Here's how the part is built. I have some questions about the finished solid (model axes, mm). A direction names the side the tool comes from. Round coordinates to 2 decimals unless told otherwise and drop trailing zeros. Order: outer loops, then holes, each group sorted by start corner. A loop starts at its lowest first (then second) coordinate and runs counter-clockwise, first axis right, second up. Notation, with made-up numbers: M 9,87.5 L 24,87.5 A18 ccw 24,122.5 Z; hole C 70.5,11 d1. An arc over 180 degrees is marked long. Use one line per item in the form item = value. Start each with the question number.
```python
from build123d import *

# Parameters (mm, degrees)
SKETCH1_W           = 12.7
SKETCH1_H           = 12.7
BOSS_EXTRUDE1_DEPTH = 2.54
FILLET1_R           = 0.635
SHELL1_START        = 0.635
SHELL1_OUTLINE_W    = 1.905
SHELL1_OUTLINE_H    = 11.43
SHELL1_DEPTH        = 11.43
SKETCH2_R           = 2.54
BOSS_EXTRUDE2_DEPTH = 1.905
BOSS_EXTRUDE3_DEPTH = 0.00254


# Read off the part's stored shape, not the designer's step: Shell1
with BuildPart() as part:
    # Sketch1 → Boss-Extrude1 (new body)
    with BuildSketch(Plane(origin=(0, 0, 0), x_dir=(1, 0, 0), z_dir=(0, 1, 0))):
        with Locations((6.35, 6.35)):
            Rectangle(SKETCH1_W, SKETCH1_H)
    extrude(amount=BOSS_EXTRUDE1_DEPTH)

    # Fillet1
    fillet1_edges = [part.edges().sort_by_distance(p)[0] for p in [
        (0, 1.27, -12.7),
        (12.7, 1.27, -12.7),
        (12.7, 1.27, 0),
        (0, 1.27, 0),
    ]]
    fillet(fillet1_edges, radius=FILLET1_R)

    # Shell1 outline → Shell1 (cut)
    with BuildSketch(Plane.YZ.offset(SHELL1_START)):
        with Locations((0.9525, -6.35)):
            Rectangle(SHELL1_OUTLINE_W, SHELL1_OUTLINE_H)
    extrude(amount=SHELL1_DEPTH, mode=Mode.SUBTRACT)

    # Sketch2 → Boss-Extrude2 (add)
    with BuildSketch(Plane(origin=(0, 1.905, 0), x_dir=(-1, 0, 0), z_dir=(0, -1, 0))):
        with Locations(Location((-6.35, 6.35, 0), (0, 0, 270))):
            Circle(SKETCH2_R)
    extrude(amount=BOSS_EXTRUDE2_DEPTH)

    # Sketch3 → Boss-Extrude3 (add)
    with BuildSketch(Plane(origin=(0, 2.54, 0), x_dir=(1, 0, 0), z_dir=(0, 1, 0))):
        Polygon((5.497146154, 8.001), (6.067017949, 8.001), (6.067017949, 6.883517027), (6.96761891, 8.001), (7.686954848, 8.001), (6.555479487, 6.596673077), (7.796985897, 4.826), (7.110722877, 4.826), (6.067017949, 6.314917268), (6.067017949, 4.826), (5.497146154, 4.826), align=None)
    extrude(amount=BOSS_EXTRUDE3_DEPTH)


solid = part.part
```
1) If we section it at C-C on z = -2.5: Write out the boundary of the cut face in (x, y) (3 decimals).
2) On a 3-axis mill with a long thin cutter (end or side, diameter ignored), from which of +Z, -Z, +X, -X, +Y, -Y can I reach the whole of each face in a straight line? I mean faces 4 (the flat face through (12.065, 1, -6)), 5 (the flat face through (0, 1, -6)). Say none if no direction works.
3) If we mould it in two halves opening along Z, with no side actions, what happens to faces 1 (the flat face through (6, 1, -12.7)), 2 (the flat face through (5, 1.905, -9)), 3 (the flat face through (5.8, 0, -0.3))? For each: +Z half, -Z half, draft (parallel to the pull), parting line (faces both ways), or undercut.
4) If we section it at D-D on z = -4: Write out the boundary of the cut face in (x, y) (3 decimals).
5) If we section it at A-A on y = 1.3: Write out the boundary of the cut face in (x, z) (3 decimals).
6) If we section it at B-B on x = 1.25: Write out the boundary of the cut face in (y, z) (3 decimals), then the cut area to 3 significant figures.
7) If I drill on line 1 (Z direction, x = 6.25, y = 0.55) (3 decimals); line 2 (Z direction, x = 11.25, y = 1.4) (3 decimals); line 3 (X direction, y = 0.4, z = -4.75) (3 decimals), over which ranges is the centre line in solid material (lowest first)?
8) Will this pin go through, and if not, where does the flat tip stop? pin 1 Ø4 at (x, z) = (3, -7.5) entering from -Y.
Completed:
q1.outline = M 0,0 L 0.635,0 L 0.635,1.905 L 12.065,1.905 L 12.065,0 L 12.7,0 L 12.7,2.54 L 0,2.54 Z
q2.face_4 = -Y
q2.face_5 = +Z, -Z, -X, +Y, -Y
q3.face_1 = -Z half
q3.face_2 = undercut
q3.face_3 = draft
q4.outline = M 0,0 L 0.635,0 L 0.635,1.905 L 5.386,1.905 L 5.386,0 L 7.314,0 L 7.314,1.905 L 12.065,1.905 L 12.065,0 L 12.7,0 L 12.7,2.54 L 0,2.54 Z
q5.outline = M 0,-12.065 A0.635 ccw 0.635,-12.7 L 12.065,-12.7 A0.635 ccw 12.7,-12.065 L 12.7,-0.635 A0.635 ccw 12.065,0 L 0.635,0 A0.635 ccw 0,-0.635 Z; C 6.35,-6.35 d5.08; hole M 0.635,-12.065 L 12.065,-12.065 L 12.065,-0.635 L 0.635,-0.635 Z
q6.outline = M 0,-12.7 L 2.54,-12.7 L 2.54,0 L 0,0 L 0,-0.635 L 1.905,-0.635 L 1.905,-12.065 L 0,-12.065 Z
q6.area = 10.5 mm²
q7.line_1 = -12.7 to -12.065, -8.888 to -3.812, -0.635 to 0
q7.line_2 = -12.7 to -12.065, -0.635 to 0
q7.line_3 = 0 to 0.635, 4.377 to 8.323, 12.065 to 12.7
q8.pin_1 = 0
